```python
from build123d import *

# Parameters (mm, degrees)
F0_W     = 63.5
F0_H     = 101.6
F0_R     = 9.525
F1_DEPTH = 25.4
F2_SIZE  = 3.175
F3_SIZE  = 1.27


with BuildPart() as f1:
    # F0 (on Top) → F1 (new body)
    with BuildSketch(Plane.XY):
        with Locations((31.75, 50.8)):
            Rectangle(F0_W, F0_H)
        with Locations((31.75, 25.4)):
            Circle(F0_R, mode=Mode.SUBTRACT)
        with Locations((31.75, 76.2)):
            Circle(F0_R, mode=Mode.SUBTRACT)
    extrude(amount=F1_DEPTH)

    # F2
    f2_edges = [f1.edges().sort_by_distance(p)[0] for p in [
        (63.5, 50.8, 25.4),
        (31.75, 101.6, 25.4),
        (0, 50.8, 25.4),
        (31.75, 0, 25.4),
    ]]
    chamfer(f2_edges, length=F2_SIZE)

    # F3
    f3_edges = [f1.edges().sort_by_distance(p)[0] for p in [
        (22.225, 76.2, 25.4),
        (22.225, 25.4, 25.4),
    ]]
    chamfer(f3_edges, length=F3_SIZE)


solid = f1.part
```
Part model, mm, in its own coordinate system. Round coordinates to 2 decimals unless told otherwise and drop trailing zeros. Loops run counter-clockwise (first coordinate to the right, second up) from the corner with the lowest first, then second, coordinate; pieces in that order, holes last.
Item 1: Mould opens along Y. For faces 1 (the face through (61.89, 50.089, 23.835)), 2 (the face through (24.191, 19.604, 11.896)), 3 (the face through (31, 101.6, 11)) say: +Y half, -Y half, draft (parallel to the pull), parting line (faces both ways), or undercut.
Item 2: Drop flat-ended pins along their axis: P1, Ø17, axis at x = 31.75, y = 76.2, coming from the -Z side; P2, Ø6, axis at x = 12, y = 87, coming from the -Z side. Give the stop position or say it passes through.
Item 3: Cut at B-B, the plane x = 31.75. Give the cut face in (y, z) (3 decimals).
Item 4: Cut at C-C, the plane z = 3.25. Give the cut face in (x, y) (3 decimals), then the cut area to 3 significant figures.
Item 5: Cut at A-A, the plane y = 25.4. Give the cut face in (x, z) (3 decimals).
Item 6: Drill centre lines: line 1 (Y direction, x = 31.75, z = 19) (3 decimals); line 2 (Y direction, x = 29, z = 17); line 3 (X direction, y = 76.5, z = 22.5) (3 decimals). Where is each one in solid material? Low to high.
A:
1. face 1: draft
1. face 2: undercut
1. face 3: +Y half
2. P1: passes through
2. P2: stops at z = 0
3. outline: (0, 0) - (15.875, 0) - (15.875, 24.13) - (14.605, 25.4) - (3.175, 25.4) - (0, 22.225) - close; (34.925, 0) - (66.675, 0) - (66.675, 24.13) - (65.405, 25.4) - (36.195, 25.4) - (34.925, 24.13) - close; (85.725, 0) - (101.6, 0) - (101.6, 22.225) - (98.425, 25.4) - (86.995, 25.4) - (85.725, 24.13) - close
4. outline: (0, 0) - (63.5, 0) - (63.5, 101.6) - (0, 101.6) - close; hole circle Ø19.05 at (31.75, 25.4); hole circle Ø19.05 at (31.75, 76.2)
4. area: 5,880 mm2
5. outline: (0, 0) - (22.225, 0) - (22.225, 24.13) - (20.955, 25.4) - (3.175, 25.4) - (0, 22.225) - close; (41.275, 0) - (63.5, 0) - (63.5, 22.225) - (60.325, 25.4) - (42.545, 25.4) - (41.275, 24.13) - close
6. line 1: y = 0 to 15.875, 34.925 to 66.675, 85.725 to 101.6
6. line 2: y = 0 to 16.28, 34.52 to 67.08, 85.32 to 101.6
6. line 3: x = 0.275 to 22.23, 41.27 to 63.225
